Build history of the part. All positions in model axes, mm. A direction names the side the tool comes from. Round coordinates to 2 decimals unless told otherwise and drop trailing zeros. Loops run counter-clockwise (first coordinate to the right, second up) from the corner with the lowest first, then second, coordinate; pieces in that order, holes last. Notation, with made-up numbers: (-38.5, 35) - (4.5, 35) arc R25 cw to (4.5, 59) - close; hole circle Ø11 at (33, -38). An arc over 180 degrees is marked (long way). Use a Markdown table: item, result.
from build123d import *

# Parameters (mm, degrees)
SKETCH2_W               = 79.375
SKETCH2_H               = 50.8
BOSS_EXTRUDE1_DEPTH     = 6.35
SKETCH3_W               = 66.675
SKETCH3_H               = 31.75
SKETCH3_W_2             = 25.4
SKETCH3_H_2             = 25.4
BOSS_EXTRUDE3_DEPTH     = 50.8
SKETCH4_W               = 25.4
SKETCH4_H               = 25.4
CUT_EXTRUDE4_DEPTH      = 7.35
CUT_EXTRUDE4_DEPTH_BACK = 58.15
SKETCH5_R               = 3.3782
CUT_EXTRUDE5_DEPTH      = 42.275
CUT_EXTRUDE6_START      = -7.35
SKETCH6_R               = 2.3876
CUT_EXTRUDE6_DEPTH      = 65.5
CIRPATTERN1_COUNT       = 4
CUT_EXTRUDE7_START      = -7.35
SKETCH7_R               = 2.3876
CUT_EXTRUDE7_DEPTH      = 65.5
CUT_EXTRUDE8_REACH      = 43.275
SKETCH9_W               = 22.225
SKETCH9_H               = 25.4
SKETCH12_W              = 12.7
SKETCH12_H              = 25.4
BOSS_EXTRUDE5_DEPTH     = 9.525
SKETCH14_W              = 12.7
SKETCH14_H              = 19.812
CUT_EXTRUDE9_DEPTH      = 6.35
SKETCH17_R              = 5.588
CUT_EXTRUDE11_DEPTH     = 6.985
BOSS_EXTRUDE6_DEPTH     = 3.81
CUT_EXTRUDE10_REACH     = 14.7
SKETCH15_R              = 1.27
SCALE1_SCALE            = 1.02


with BuildPart() as part:
    # Sketch2 → Boss-Extrude1 (new body)
    with BuildSketch(Plane(origin=(0, 0, 0), x_dir=(1, 0, 0), z_dir=(0, 1, 0))):
        Rectangle(SKETCH2_W, SKETCH2_H)
    boss_extrude1 = extrude(amount=BOSS_EXTRUDE1_DEPTH)

    # Sketch3 → Boss-Extrude3 (add)
    with BuildSketch(Plane(origin=(0, 6.35, 0), x_dir=(1, 0, 0), z_dir=(0, 1, 0))):
        with Locations((-3.175, 0)):
            Rectangle(SKETCH3_W, SKETCH3_H)
        with Locations((-20.6375, 0)):
            Rectangle(SKETCH3_W_2, SKETCH3_H_2, mode=Mode.SUBTRACT)
        with Locations((14.2875, 0)):
            Rectangle(SKETCH3_W_2, SKETCH3_H_2, mode=Mode.SUBTRACT)
    extrude(amount=BOSS_EXTRUDE3_DEPTH)

    # Mirror1: Boss-Extrude1 across plane
    add(boss_extrude1.mirror(Plane.ZX.offset(31.75)))

    # Sketch4 → Cut-Extrude4 (cut, two sides)
    with BuildSketch(Plane(origin=(0, 57.15, 0), x_dir=(1, 0, 0), z_dir=(0, 1, 0))) as cut_extrude4_sk:
        with Locations((-20.6375, 0)):
            Rectangle(SKETCH4_W, SKETCH4_H)
        with Locations((14.2875, 0)):
            Rectangle(SKETCH4_W, SKETCH4_H)
    extrude(amount=CUT_EXTRUDE4_DEPTH, mode=Mode.SUBTRACT)
    extrude(cut_extrude4_sk.sketch, amount=-CUT_EXTRUDE4_DEPTH_BACK, mode=Mode.SUBTRACT)

    # Sketch5 → Cut-Extrude5 (cut, through all)
    with BuildSketch(Plane.XY.offset(15.875)):
        with Locations((-20.6375, 31.75)):
            Circle(SKETCH5_R)
    extrude(amount=-CUT_EXTRUDE5_DEPTH, mode=Mode.SUBTRACT)

    # Sketch6 → Cut-Extrude6 (cut)
    with BuildSketch(Plane(origin=(0, 6.35, 0), x_dir=(1, 0, 0), z_dir=(0, 1, 0)).offset(CUT_EXTRUDE6_START)):
        with Locations((34.925, 0)):
            Circle(SKETCH6_R)
    cut_extrude6 = extrude(amount=CUT_EXTRUDE6_DEPTH, mode=Mode.SUBTRACT)

    # CirPattern1: Cut-Extrude6 ×4 about axis, 1 skipped
    cirpattern1_axis = Axis((14.2875, 0, 0), (0, 1, 0))
    add([cut_extrude6.rotate(cirpattern1_axis, i * 360 / CIRPATTERN1_COUNT) for i in range(1, CIRPATTERN1_COUNT) if i not in (2,)], mode=Mode.SUBTRACT)

    # Sketch7 → Cut-Extrude7 (cut)
    with BuildSketch(Plane(origin=(0, 6.35, 0), x_dir=(1, 0, 0), z_dir=(0, 1, 0)).offset(CUT_EXTRUDE7_START)):
        with Locations((-20.6375, -20.6375)):
            Circle(SKETCH7_R)
    cut_extrude7 = extrude(amount=CUT_EXTRUDE7_DEPTH, mode=Mode.SUBTRACT)

    # Mirror2: Cut-Extrude7 across plane
    add(cut_extrude7.mirror(Plane.XY), mode=Mode.SUBTRACT)

    # Sketch9 → Cut-Extrude8 (cut, up to next)
    with BuildSketch(Plane(origin=(0, 0, -15.875), x_dir=(-1, 0, 0), z_dir=(0, 0, -1)), mode=Mode.PRIVATE) as cut_extrude8_sk1:
        with Locations((-12.7, 19.05)):
            Rectangle(SKETCH9_W, SKETCH9_H)
    cut_extrude8_tool1 = extrude(cut_extrude8_sk1.sketch, amount=-CUT_EXTRUDE8_REACH, mode=Mode.PRIVATE) & part.part
    add(cut_extrude8_tool1.solids().sort_by_distance((12.7, 19.05, -15.875))[0], mode=Mode.SUBTRACT)

    # Sketch12 → Boss-Extrude5 (add)
    with BuildSketch(Plane(origin=(30.1625, 0, 0), x_dir=(0, 0, -1), z_dir=(1, 0, 0))):
        with Locations((19.05, 19.05)):
            Rectangle(SKETCH12_W, SKETCH12_H)
    extrude(amount=-BOSS_EXTRUDE5_DEPTH)

    # Sketch14 → Cut-Extrude9 (cut)
    with BuildSketch(Plane.ZY.offset(-20.6375)):
        with Locations((-19.05, 16.256)):
            Rectangle(SKETCH14_W, SKETCH14_H)
    extrude(amount=-CUT_EXTRUDE9_DEPTH, mode=Mode.SUBTRACT)

    # Sketch17 → Cut-Extrude11 (cut)
    with BuildSketch(Plane.ZY.offset(-26.9875)):
        with Locations((-12.7, 26.123322238)):
            Circle(SKETCH17_R)
    extrude(amount=CUT_EXTRUDE11_DEPTH, mode=Mode.SUBTRACT)

    # Sketch19 → Boss-Extrude6 (add)
    with BuildSketch(Plane(origin=(0, 0, -25.4), x_dir=(-1, 0, 0), z_dir=(0, 0, -1))):
        Polygon((-26.9875, 26.162), (-20.6375, 26.162), (-20.6375, 31.75), (-30.1625, 31.75), (-30.1625, 6.35), (-39.6875, 6.35), (-39.6875, 0), (-20.6375, 0), (-20.6375, 6.35), (-26.9875, 6.35), align=None)
    extrude(amount=BOSS_EXTRUDE6_DEPTH)

    # Sketch15 → Cut-Extrude10 (cut, up to next)
    with BuildSketch(Plane.ZY.offset(-26.9875), mode=Mode.PRIVATE) as cut_extrude10_sk1:
        with BuildLine():
            Line((-24.3078, 12.954), (-25.5778, 12.954))
            ThreePointArc((-25.5778, 12.954), (-24.679774388, 12.582025612), (-24.3078, 11.684))
            ThreePointArc((-24.3078, 11.684), (-24.679774388, 10.785974388), (-25.5778, 10.414))
            Line((-25.5778, 10.414), (-24.3078, 10.414))
            ThreePointArc((-24.3078, 10.414), (-23.0378, 11.684), (-24.3078, 12.954))
        make_face()
    cut_extrude10_tool1 = extrude(cut_extrude10_sk1.sketch, amount=-CUT_EXTRUDE10_REACH, mode=Mode.PRIVATE) & part.part
    add(cut_extrude10_tool1.solids().sort_by_distance((26.9875, 11.684, -23.945344))[0], mode=Mode.SUBTRACT)
    # Sketch15 → Cut-Extrude10 (cut, up to next)
    with BuildSketch(Plane.ZY.offset(-26.9875), mode=Mode.PRIVATE) as cut_extrude10_sk2:
        with BuildLine():
            Line((-25.5778, 12.954), (-26.8478, 12.954))
            ThreePointArc((-26.8478, 12.954), (-28.1178, 11.684), (-26.8478, 10.414))
            Line((-26.8478, 10.414), (-25.5778, 10.414))
            ThreePointArc((-25.5778, 10.414), (-26.8478, 11.684), (-25.5778, 12.954))
        make_face()
    cut_extrude10_tool2 = extrude(cut_extrude10_sk2.sketch, amount=-CUT_EXTRUDE10_REACH, mode=Mode.PRIVATE) & part.part
    add(cut_extrude10_tool2.solids().sort_by_distance((26.9875, 11.684, -27.210256))[0], mode=Mode.SUBTRACT)
    # Sketch15 → Cut-Extrude10 (cut, up to next)
    with BuildSketch(Plane.ZY.offset(-26.9875), mode=Mode.PRIVATE) as cut_extrude10_sk3:
        with Locations((-25.5778, 11.684)):
            Circle(SKETCH15_R)
    cut_extrude10_tool3 = extrude(cut_extrude10_sk3.sketch, amount=-CUT_EXTRUDE10_REACH, mode=Mode.PRIVATE) & part.part
    add(cut_extrude10_tool3.solids().sort_by_distance((26.9875, 11.684, -25.5778))[0], mode=Mode.SUBTRACT)
    # Sketch15 → Cut-Extrude10 (cut, up to next)
    with BuildSketch(Plane.ZY.offset(-26.9875), mode=Mode.PRIVATE) as cut_extrude10_sk4:
        with BuildLine():
            Line((-24.3078, 22.606), (-25.5778, 22.606))
            ThreePointArc((-25.5778, 22.606), (-24.679774388, 22.234025612), (-24.3078, 21.336))
            ThreePointArc((-24.3078, 21.336), (-24.679774388, 20.437974388), (-25.5778, 20.066))
            Line((-25.5778, 20.066), (-24.3078, 20.066))
            ThreePointArc((-24.3078, 20.066), (-23.0378, 21.336), (-24.3078, 22.606))
        make_face()
    cut_extrude10_tool4 = extrude(cut_extrude10_sk4.sketch, amount=-CUT_EXTRUDE10_REACH, mode=Mode.PRIVATE) & part.part
    add(cut_extrude10_tool4.solids().sort_by_distance((26.9875, 21.336, -23.945344))[0], mode=Mode.SUBTRACT)
    # Sketch15 → Cut-Extrude10 (cut, up to next)
    with BuildSketch(Plane.ZY.offset(-26.9875), mode=Mode.PRIVATE) as cut_extrude10_sk5:
        with Locations((-25.5778, 21.336)):
            Circle(SKETCH15_R)
    cut_extrude10_tool5 = extrude(cut_extrude10_sk5.sketch, amount=-CUT_EXTRUDE10_REACH, mode=Mode.PRIVATE) & part.part
    add(cut_extrude10_tool5.solids().sort_by_distance((26.9875, 21.336, -25.5778))[0], mode=Mode.SUBTRACT)
    # Sketch15 → Cut-Extrude10 (cut, up to next)
    with BuildSketch(Plane.ZY.offset(-26.9875), mode=Mode.PRIVATE) as cut_extrude10_sk6:
        with BuildLine():
            Line((-25.5778, 22.606), (-26.8478, 22.606))
            ThreePointArc((-26.8478, 22.606), (-28.1178, 21.336), (-26.8478, 20.066))
            Line((-26.8478, 20.066), (-25.5778, 20.066))
            ThreePointArc((-25.5778, 20.066), (-26.8478, 21.336), (-25.5778, 22.606))
        make_face()
    cut_extrude10_tool6 = extrude(cut_extrude10_sk6.sketch, amount=-CUT_EXTRUDE10_REACH, mode=Mode.PRIVATE) & part.part
    add(cut_extrude10_tool6.solids().sort_by_distance((26.9875, 21.336, -27.210256))[0], mode=Mode.SUBTRACT)


with BuildPart() as part_1:
    # Scale1: scaled about (-0.77165693, 31.73889904, -0.207713898)
    add(part.part.scale(SCALE1_SCALE).moved(Location((0.015433139, -0.634777981, 0.004154278))))


solid = part_1.part
Q1. Drop flat-ended pins along their axis: pin 1 (3 mm diameter, centred on x = -19, y = 3, fed in from -Z); pin 2 (13 mm diameter, centred on y = 30.5, z = 0, fed in from -X); pin 3 (16.5 mm diameter, centred on x = -16, z = -2.5, fed in from +Y); pin 4 (3 mm diameter, centred on y = 24, z = -22, fed in from +X). Give the stop position or say it passes through.
Results found:
| item | result |
|---|---|
| pin 1 | stops at z = -25.9 |
| pin 2 | stops at x = -37.23 |
| pin 3 | stops at y = 64.14 |
| pin 4 | stops at x = 30.78 |
Q2. Probe line 1 (X direction, y = 49, z = -2); line 2 (X direction, y = 5.5, z = 11); line 3 (Z direction, x = -29.5, y = 44.5). List the from-to ranges inside material, lowest first.
Results found:
| item | result |
|---|---|
| line 1 | x = -37.23 to -33.99, -8.08 to 1.63, 27.54 to 30.78 |
| line 2 | x = -40.47 to -33.99, -8.08 to 1.63, 27.54 to 40.5 |
| line 3 | z = -16.19 to -12.95, 12.96 to 16.2 |
Q3. Cut at B-B, the plane x = 4. List the corners of the cut face in (y, z).
Results found:
| item | result |
|---|---|
| outline | (-0.63, -25.9) - (5.84, -25.9) - (5.84, -12.95) - (-0.63, -12.95) - close; (-0.63, 12.96) - (64.14, 12.96) - (64.14, 25.91) - (57.66, 25.91) - (57.66, 16.2) - (5.84, 16.2) - (5.84, 25.91) - (-0.63, 25.91) - close; (31.75, -16.19) - (57.66, -16.19) - (57.66, -25.9) - (64.14, -25.9) - (64.14, -12.95) - (31.75, -12.95) - close |
Q4. Cut at C-C, the plane y = 48.5. List the corners of the cut face in (x, z), plus the area to 3 significant figures.
Results found:
| item | result |
|---|---|
| outline | (-37.23, -16.19) - (30.78, -16.19) - (30.78, 16.2) - (-37.23, 16.2) - close; hole (-33.99, -12.95) - (-8.08, -12.95) - (-8.08, 12.96) - (-33.99, 12.96) - close; hole (1.63, -12.95) - (27.54, -12.95) - (27.54, 12.96) - (1.63, 12.96) - close |
| area | 860 mm2 |
Q5. Which spindle directions (+Z, -Z, +X, -X, +Y, -Y) get a long thin tool onto all of the face, cutting with end or side? Do faces 1 (the face through (-4, 31, 16.197)), 2 (the face through (24, 26.05, -24)), 3 (the face through (11, 31.75, -15)), 4 (the face through (21.066, 3, -28)). Say none if no direction does.
Results found:
| item | result |
|---|---|
| face 1 | +Z, +X, -X |
| face 2 | -Z, -X |
| face 3 | -Z |
| face 4 | -Z, -X, +Y, -Y |
Q6. Cut at D-D, the plane x = 22.5. List the corners of the cut face in (y, z), plus the area to 3 significant figures.
Results found:
| item | result |
|---|---|
| outline | (-0.63, -29.79) - (5.84, -29.79) - (5.84, -12.95) - (-0.63, -12.95) - close; (-0.63, 12.96) - (64.14, 12.96) - (64.14, 25.91) - (57.66, 25.91) - (57.66, 16.2) - (5.84, 16.2) - (5.84, 25.91) - (-0.63, 25.91) - close; (26.05, -29.79) - (31.75, -29.79) - (31.75, -16.19) - (57.66, -16.19) - (57.66, -25.9) - (64.14, -25.9) - (64.14, -12.95) - (31.71, -12.95) arc R5.7 cw to (26.05, -18.65) - close |
| area | 683 mm2 |
Q7. Cut at A-A, the plane z = -11. List the corners of the cut face in (x, y), plus the area to 3 significant figures.
Results found:
| item | result |
|---|---|
| outline | (-40.47, -0.63) - (-33.99, -0.63) - (-33.99, 64.14) - (-40.47, 64.14) - (-40.47, 57.66) - (-37.23, 57.66) - (-37.23, 5.84) - (-40.47, 5.84) - close; (-8.08, -0.63) - (1.63, -0.63) - (1.63, 64.14) - (-8.08, 64.14) - close; (27.54, -0.63) - (40.5, -0.63) - (40.5, 5.84) - (30.78, 5.84) - (30.78, 57.66) - (40.5, 57.66) - (40.5, 64.14) - (27.54, 64.14) - close |
| area | 1,220 mm2 |
Q8. Pull direction Z, two halves, no side cores. Call faces 5 (the face through (-21.35, 60.85, 18.64)), 6 (the face through (-1, 61, -25.904)), 7 (the face through (26, 31.75, -23)), 8 (the face through (-1, 61, 25.912)): pulls with the +Z half, pulls with the -Z half, needs draft (parallel to the pull), parting line crosses it, or undercut.
Results found:
| item | result |
|---|---|
| face 5 | undercut |
| face 6 | pulls with the -Z half |
| face 7 | needs draft |
| face 8 | pulls with the +Z half |
